```python
from build123d import *

# Parameters (mm, degrees)
F0_W           = 254
F0_H           = 90
F0_R           = 6
F1_DEPTH       = 3
F3_D           = 3.5
F3_CBORE_D     = 6.5
F3_CBORE_DEPTH = 2
F4_R           = 2


with BuildPart() as f1:
    # F0 (on Front) → F1 (new body)
    with BuildSketch(Plane.XZ):
        Rectangle(F0_W, F0_H)
        with Locations((-97, 0)):
            Circle(F0_R, mode=Mode.SUBTRACT)
        with BuildLine():
            Line((-44, -3), (-44, 3))
            ThreePointArc((-44, 3), (-40, 5), (-36, 3))
            Line((-36, 3), (-36, -3))
            ThreePointArc((-36, -3), (-40, -5), (-44, -3))
        make_face(mode=Mode.SUBTRACT)
        with BuildLine():
            ThreePointArc((44.814302, -1.35), (35, 0), (44.814302, 1.35))
            Line((44.814302, 1.35), (47.5, 1.35))
            Line((47.5, 1.35), (47.5, -1.35))
            Line((47.5, -1.35), (44.814302, -1.35))
        make_face(mode=Mode.SUBTRACT)
        with Locations((97, 0)):
            Circle(F0_R, mode=Mode.SUBTRACT)
    extrude(amount=F1_DEPTH)

    # F3 (through all)
    with Locations(Plane.XZ.offset(3)):
        with Locations((-122, 40), (-122, -40), (122, 40), (122, -40)):
            CounterBoreHole(F3_D / 2, F3_CBORE_D / 2, F3_CBORE_DEPTH)

    # F4
    f4_edges = [f1.edges().sort_by_distance(p)[0] for p in [
        (-127, -1.5, 45),
        (-127, -1.5, -45),
        (127, -1.5, -45),
        (127, -1.5, 45),
    ]]
    fillet(f4_edges, radius=F4_R)


solid = f1.part
```
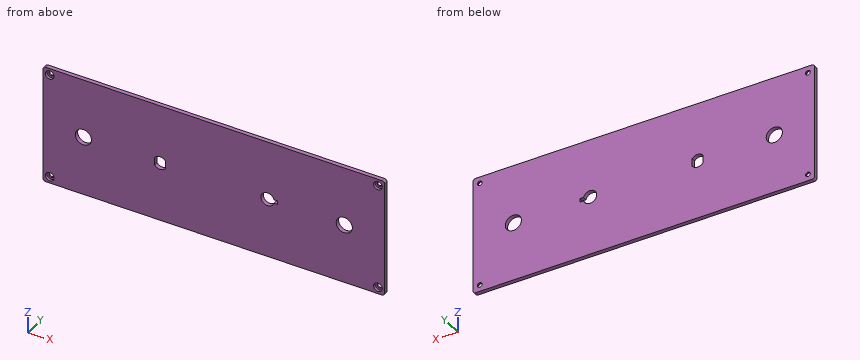
Geometry: final body of the model. Coordinates: model frame, mm. Round coordinates to 2 decimals unless told otherwise and drop trailing zeros. Order: outer loops, then holes, each group sorted by start corner. A loop starts at its lowest first (then second) coordinate and runs counter-clockwise, first axis right, second up. Notation, with made-up numbers: (3.25, 34.25) -> (31.25, 34.25) arc R18 cw to (31.25, 52.25) -> close; hole circle Ø2 at (29.25, -9.5). An arc over 180 degrees is marked (long way). Use CSV: the item, a comma, the result in double quotes. Start each with the question number.
1) First-contact query: pin 1 Ø4.5 at (x, z) = (122, -40) entering from -Y; pin 2 Ø3 at (x, z) = (122, 40) entering from -Y. Flat tips, straight axial feed; report the tip coordinate or a pass-through.
2) Section B-B (y = -0.45). State how many separate pieces and enclosed holes the cut face has, and give its area (3 significant figures).
3) Section A-A (x = 97). Return the cut outline in (y, z), and give its area (3 significant figures).
4) Section C-C (x = 40). Return the cut outline in (y, z), and give its area (3 significant figures).
5) Material intervals for line 1 along Z through (x, y) = (40, -1); line 2 along Z through (x, y) = (122, -0.8); line 3 along Z through (x, y) = (-122, -1.5), sorted ascending. Write a range as from..to.
Returned:
1,pin 1,"stops at y = -1"
1,pin 2,"passes through"
2,separate pieces,"1"
2,enclosed holes,"8"
2,area,"22,400 mm²"
3,outline,"(-3, -45) -> (0, -45) -> (0, -6) -> (-3, -6) -> close; (-3, 6) -> (0, 6) -> (0, 45) -> (-3, 45) -> close"
3,area,"234 mm²"
4,outline,"(-3, -45) -> (0, -45) -> (0, -5) -> (-3, -5) -> close; (-3, 5) -> (0, 5) -> (0, 45) -> (-3, 45) -> close"
4,area,"240 mm²"
5,line 1,"z = -45..-5, 5..45"
5,line 2,"z = -45..-41.75, -38.25..38.25, 41.75..45"
5,line 3,"z = -45..-43.25, -36.75..36.75, 43.25..45"
